```python
from build123d import *

# Parameters (mm, degrees)
SKETCH1_W           = 5
SKETCH1_H           = 20
SKETCH1_H_2         = 5
SKETCH1_W_2         = 25
BOSS_EXTRUDE1_DEPTH = 12
SKETCH2_R           = 2.2
CUT_EXTRUDE1_DEPTH  = 12
CUT_EXTRUDE3_DEPTH  = 5


with BuildPart() as part:
    # Sketch1 → Boss-Extrude1 (new body)
    with BuildSketch(Plane(origin=(0, 0, 0), x_dir=(0, 0, -1), z_dir=(1, 0, 0))):
        with Locations((2.5, 15)):
            Rectangle(SKETCH1_W, SKETCH1_H)
        with Locations((2.5, 2.5)):
            Rectangle(SKETCH1_W, SKETCH1_H_2)
        with Locations((17.5, 2.5)):
            Rectangle(SKETCH1_W_2, SKETCH1_H_2)
    extrude(amount=BOSS_EXTRUDE1_DEPTH)

    # Sketch2 → Cut-Extrude1 (cut)
    with BuildSketch(Plane(origin=(0, 0, -5), x_dir=(-1, 0, 0), z_dir=(0, 0, -1))):
        with Locations((-6, 19.75)):
            Circle(SKETCH2_R)
        with Locations((-6, 9.75)):
            Circle(SKETCH2_R)
    extrude(amount=-CUT_EXTRUDE1_DEPTH, mode=Mode.SUBTRACT)

    # Sketch3 → Cut-Extrude3 (cut)
    with BuildSketch(Plane.XZ):
        with BuildLine():
            ThreePointArc((8.2, -25), (7.555634919, -23.444365081), (6, -22.8))
            Line((6, -22.8), (6, -27.2))
            ThreePointArc((6, -27.2), (7.555634919, -26.555634919), (8.2, -25))
        make_face()
        with BuildLine():
            Line((6, -27.2), (6, -22.8))
            ThreePointArc((6, -22.8), (3.8, -25), (6, -27.2))
        make_face()
    extrude(amount=-CUT_EXTRUDE3_DEPTH, mode=Mode.SUBTRACT)


solid = part.part
```
The model under review builds one solid part; all positions refer to its coordinate system, in mm. A direction names the side the tool comes from. Coordinates: 2 decimals unless noted, no trailing zeros. Write each loop counter-clockwise with the first axis right and the second up, starting at its lowest first coordinate (ties: lowest second). Pieces come first, ordered by that corner, then holes. Notation, with made-up numbers: (-30.5, 59) - (-5.5, 59) arc R18 ccw to (-5.5, 94) - close; hole circle Ø3 at (3, -21). An arc over 180 degrees is marked (long way). Answer in a Markdown table with one row per item. Add a question column.
Q1. Draft analysis for pull direction Y (two halves, no side actions). For faces 1 (the face through (6, 5, -17)), 2 (the face through (6, 2, -30)), 3 (the face through (4.98, 17.8, -2.54)), state which applies: +Y half, -Y half, draft (parallel to the pull), parting line (faces both ways), or undercut.
Q2. To check wall thickness, follow line 1 along Y through (x, z) = (6, -3.8); line 2 along Z through (x, y) = (6.25, 14.75); line 3 along Y through (x, z) = (3.75, -11.75). State the ranges of each line that lie inside material, in increasing order. Write a range as from..to.
Q3. Consider section D-D on z = -19.25. Give the boundary of the cut face in (x, y), then the cut area to 3 significant figures.
Q4. Clearance check with flat-ended pins moving along their axes: pin 1 (3.5 mm diameter, centred on x = 9, z = -13.5, fed in from +Y); pin 2 (1 mm diameter, centred on x = 5, y = 12.5, fed in from -Z). State where each tip first meets the part, or that it passes through.
Q5. Consider section B-B on z = -4.25. Give the boundary of the cut face in (x, y).
Q6. For faces 4 (the face through (6, 15, -5)), 5 (the face through (3.9, 10.4, -2.5)), list the 3-axis set-ups (+Z, -Z, +X, -X, +Y, -Y) from which the entire face can be reached by the end or side of a thin tool; tool diameter is ignored.
Q7. Consider section A-A on y = 19.75. Give the boundary of the cut face in (x, z).
Q8. Consider section C-C on x = 11. Give the boundary of the cut face in (y, z).
Answers below:
| question | item | result |
|---|---|---|
| 1 | face 1 | +Y half |
| 1 | face 2 | draft |
| 1 | face 3 | undercut |
| 2 | line 1 | 0..7.55, 11.95..17.55, 21.95..25 |
| 2 | line 2 | -5..0 |
| 2 | line 3 | 0..5 |
| 3 | outline | (0, 0) - (12, 0) - (12, 5) - (0, 5) - close |
| 3 | area | 60.0 mm² |
| 4 | pin 1 | y = 5 |
| 4 | pin 2 | z = -5 |
| 5 | outline | (0, 0) - (12, 0) - (12, 25) - (0, 25) - close; hole circle Ø4.4 at (6, 9.75); hole circle Ø4.4 at (6, 19.75) |
| 6 | face 4 | -Z, +X, -X, +Y |
| 6 | face 5 | +Z, -Z |
| 7 | outline | (0, -5) - (3.8, -5) - (3.8, 0) - (0, 0) - close; (8.2, -5) - (12, -5) - (12, 0) - (8.2, 0) - close |
| 8 | outline | (0, -30) - (5, -30) - (5, -5) - (25, -5) - (25, 0) - (0, 0) - close |
